```python
from build123d import *

# Parameters (mm, degrees)
SK_P02_MODULEPLATE_W  = 24
SK_P02_MODULEPLATE_H  = 5
P02_MODULEPLATE_DEPTH = 40
SK_P03_MODULEPLATE_W  = 24
SK_P03_MODULEPLATE_H  = 5
P03_MODULEPLATE_DEPTH = 36
P04_TRAILINGARM_START = 22
SK_P04_TRAILINGARM_W  = 50
SK_P04_TRAILINGARM_H  = 5
P04_TRAILINGARM_DEPTH = 16
P05_PIVOTBOSS_START   = 31
SK_P05_PIVOTBOSS_R    = 9
P05_PIVOTBOSS_DEPTH   = 5
P06_SPRINGTAB_START   = 21
SK_P06_SPRINGTAB_W    = 16
SK_P06_SPRINGTAB_H    = 31
P06_SPRINGTAB_DEPTH   = 4


with BuildPart() as part:
    # SK_P01_Gearmotor37Dwith64CPRenc → P01_Gearmotor37Dwith64CPRenc (revolve)
    with BuildSketch(Plane(origin=(0, 20.5, 0), x_dir=(1, 0, 0), z_dir=(0, 1, 0)), mode=Mode.PRIVATE) as p01_gearmotor37dwith64cprenc_sk:
        Polygon((17.5, -49), (20.5, -49), (20.5, -31), (36, -31), (36, 7), (35, 7), (35, 39), (33.5, 39), (33.5, 49), (17.5, 49), align=None)
    revolve(p01_gearmotor37dwith64cprenc_sk.sketch.rotate(Axis((17.5, 20.5, -54), (0, 0, 1)), 180), axis=Axis((17.5, 20.5, -54), (0, 0, 1)))

    # SK_P02_Moduleplate → P02_Moduleplate (add)
    with BuildSketch(Plane(origin=(0, 0, 0), x_dir=(1, 0, 0), z_dir=(0, 1, 0))):
        with Locations((5.5, -33.5)):
            Rectangle(SK_P02_MODULEPLATE_W, SK_P02_MODULEPLATE_H)
    extrude(amount=P02_MODULEPLATE_DEPTH)

    # SK_P03_Moduleplate → P03_Moduleplate (add)
    with BuildSketch(Plane(origin=(0, 0, 0), x_dir=(1, 0, 0), z_dir=(0, 1, 0))):
        with Locations((29.5, -33.5)):
            Rectangle(SK_P03_MODULEPLATE_W, SK_P03_MODULEPLATE_H)
    extrude(amount=P03_MODULEPLATE_DEPTH)

    # SK_P04_Trailingarm → P04_Trailingarm (add)
    with BuildSketch(Plane(origin=(0, 0, 0), x_dir=(1, 0, 0), z_dir=(0, 1, 0)).offset(P04_TRAILINGARM_START)):
        with Locations((-31.5, -33.5)):
            Rectangle(SK_P04_TRAILINGARM_W, SK_P04_TRAILINGARM_H)
    extrude(amount=P04_TRAILINGARM_DEPTH)

    # SK_P05_Pivotboss → P05_Pivotboss (add)
    with BuildSketch(Plane.XY.offset(P05_PIVOTBOSS_START)):
        with Locations((-48.5, 30)):
            Circle(SK_P05_PIVOTBOSS_R)
    extrude(amount=P05_PIVOTBOSS_DEPTH)

    # SK_P06_Springtab → P06_Springtab (add)
    with BuildSketch(Plane(origin=(0, 0, 0), x_dir=(1, 0, 0), z_dir=(0, 1, 0)).offset(P06_SPRINGTAB_START)):
        with Locations((49.5, -20.5)):
            Rectangle(SK_P06_SPRINGTAB_W, SK_P06_SPRINGTAB_H)
    extrude(amount=P06_SPRINGTAB_DEPTH)


solid = part.part
```
Geometry: final body of the model. Coordinates: model frame, mm. A direction names the side the tool comes from. Coordinates: 2 decimals unless noted, no trailing zeros. Loops run counter-clockwise (first coordinate to the right, second up) from the corner with the lowest first, then second, coordinate; pieces in that order, holes last. Notation, with made-up numbers: M 15,-10.75 L 30,-10.75 A28 cw 30,18.25 Z; hole C 39.5,-39.5 d11. An arc over 180 degrees is marked long. Put each result on its own line as item: value.
(1) Cut plane A-A on z = 19.5. Return the cut outline in (x, y), then the cut area to 3 significant figures.
Answer sheet:
outline: C 17.5,20.5 d37; M 41.5,21 L 57.5,21 L 57.5,25 L 41.5,25 Z
area: 1,140 mm^2
(2) Draft query along X for faces 4 (the face through (41.5, 23, 18)), 5 (the face through (41.5, 30, 34)), 6 (the face through (-26, 38, 33)), 7 (the face through (21, 37, 31)). Return one class per face: pulls with the +X half, pulls with the -X half, needs draft (parallel to the pull), parting line crosses it, or undercut.
Answer sheet:
face 4: undercut
face 5: pulls with the +X half
face 6: undercut
face 7: needs draft
(3) Material intervals for probe 1 along Z at (x, y) = (-22.5, 31.5); probe 2 along Z at (x, y) = (14, 3.5); probe 3 along Y at (x, z) = (16.5, 6.5), sorted ascending.
Answer sheet:
probe 1: z = 31 to 36
probe 2: z = -39 to 36
probe 3: y = 2.03 to 38.97
(4) Access query for faces 1 (the face through (-9, 24, 31)), 2 (the face through (29, 36, 33)), 3 (the face through (49, 25, 20)). Directions: +Z, -Z, +X, -X, +Y, -Y. A direction counts if a zero-diameter tool reaches every point of the face in a straight line with its end or side. Return the directions, or none.
Answer sheet:
face 1: -Z
face 2: +Z, +X, +Y
face 3: +Z, -Z, +X, +Y
(5) Cut plane D-D on z = -23.5. Return the cut outline in (x, y).
Answer sheet:
outline: C 17.5,20.5 d35
(6) Cut plane B-B on y = 12. Return the cut outline in (x, z).
Answer sheet:
outline: M -6.5,31 L 1.07,31 L 1.07,-7 L 2.2,-7 L 2.2,-39 L 3.94,-39 L 3.94,-49 L 31.06,-49 L 31.06,-39 L 32.8,-39 L 32.8,-7 L 33.93,-7 L 33.93,31 L 41.5,31 L 41.5,36 L -6.5,36 Z
(7) Cut plane C-C on x = 19. Return the cut outline in (y, z).
Answer sheet:
outline: M 0,31 L 2.06,31 L 2.06,-7 L 3.06,-7 L 3.06,-39 L 4.57,-39 L 4.57,-49 L 36.43,-49 L 36.43,-39 L 37.94,-39 L 37.94,-7 L 38.94,-7 L 38.94,31 L 36,31 L 36,36 L 23.1,36 L 23.1,49 L 17.9,49 L 17.9,36 L 0,36 Z
(8) First-contact query: pin 1 (8 mm diameter, centred on y = 30.5, z = -16, fed in from -X); pin 2 (4 mm diameter, centred on y = 30.5, z = 33.5, fed in from +X); pin 3 (6 mm diameter, centred on y = 15, z = 22.5, fed in from -X). Flat tips, straight axial feed; report the tip coordinate or a pass-through.
Answer sheet:
pin 1: stops at x = 1.06
pin 2: stops at x = 41.5
pin 3: stops at x = -0.83
